from build123d import *

# Parameters (mm, degrees)
F1_DEPTH = 60.325
F2_R     = 6.35
F3_R     = 6.35
F4_W     = 17.4625
F4_H     = 17.4625
F5_DEPTH = 25.4


with BuildPart() as f1:
    # F0 (on Front) → F1 (new body)
    with BuildSketch(Plane.XZ):
        with BuildLine():
            ThreePointArc((18.421305, 15.875), (-31.178134, 43.737725), (-67.557349, 0))
            Line((-67.557349, 0), (-51.682349, 0))
            ThreePointArc((-51.682349, 0), (-23.107349, 28.575), (5.467651, 0))
            Line((5.467651, 0), (65.792651, 0))
            Line((65.792651, 0), (65.792651, 57.15))
            Line((65.792651, 57.15), (49.917651, 57.15))
            Line((49.917651, 57.15), (49.917651, 15.875))
            Line((49.917651, 15.875), (18.421305, 15.875))
        make_face()
    extrude(amount=F1_DEPTH)

    # F2
    f2_edges = [f1.edges().sort_by_distance(p)[0] for p in [
        (57.855151, -60.325, 57.15),
    ]]
    fillet(f2_edges, radius=F2_R)

    # F3
    f3_edges = [f1.edges().sort_by_distance(p)[0] for p in [
        (57.855151, 0, 57.15),
    ]]
    fillet(f3_edges, radius=F3_R)

    # F4 (on face) → F5 (cut)
    with BuildSketch(Plane.YZ.offset(65.792651)):
        with Locations((-31.080982, 48.41875)):
            Rectangle(F4_W, F4_H)
        with BuildLine():
            Line((-22.349732, 39.6875), (-39.812232, 39.6875))
            ThreePointArc((-39.812232, 39.6875), (-31.080982, 30.95625), (-22.349732, 39.6875))
        make_face()
    extrude(amount=-F5_DEPTH, mode=Mode.SUBTRACT)


solid = f1.part
Check sheet for the modelled part. Datum: model origin and axes. Units: mm. A direction names the side the tool comes from. Round coordinates to 2 decimals unless told otherwise and drop trailing zeros. Write each loop counter-clockwise with the first axis right and the second up, starting at its lowest first coordinate (ties: lowest second). Pieces come first, ordered by that corner, then holes. Notation, with made-up numbers: (35.25, -6.5) - (65.25, -6.5) arc R11 cw to (65.25, 12.5) - close; hole circle Ø8 at (78, 74). An arc over 180 degrees is marked (long way). Return JSON: item names as keys, results as strings.
Q1. Cross-section at B-B (y = -44). Record the boundary of the cut face in (x, z) (3 decimals), then the cut area to 3 significant figures.
Returned:
{"outline": "(-67.557, 0) - (-51.682, 0) arc R28.575 cw to (5.468, 0) - (65.793, 0) - (65.793, 57.15) - (49.918, 57.15) - (49.918, 15.875) - (18.421, 15.875) arc R44.45 ccw to start", "area": "3,200 mm²"}
Q2. Draft check along Y on faces 1 (the cylindrical face through (57.74, -1.91, 55.34)), 2 (the cylindrical face through (57.744, -58.415, 55.339)), 3 (the flat face through (58, -39.812, 48)), 4 (the flat face through (35, -30, 0)). Enter one of: released by +Y, released by -Y, zero draft, split by the parting line, or undercut.
Returned:
{"face 1": "released by +Y", "face 2": "released by -Y", "face 3": "undercut", "face 4": "zero draft"}
Q3. Depth check by flat-ended pin: P1, Ø3, axis at x = -34.5, z = 26, coming from the +Y side; P2, Ø4, axis at y = -36, z = 9, coming from the -X side; P3, Ø5, axis at x = -53, y = -34, coming from the +Z side; P4, Ø10, axis at y = -53.5, z = 20, coming from the -X side. Enter the tip coordinate at first touch or a pass-through.
Returned:
{"P1": "stops at y = 0", "P2": "stops at x = -67.01", "P3": "stops at z = 35.03", "P4": "stops at x = -64.96"}
Q4. Cross-section at A-A (z = 48.5). Record the boundary of the cut face in (x, y) (3 decimals), then the cut area to 3 significant figures.
Returned:
{"outline": "(49.918, -60.325) - (65.793, -60.325) - (65.793, -39.812) - (49.918, -39.812) - close; (49.918, -22.35) - (65.793, -22.35) - (65.793, 0) - (49.918, 0) - close", "area": "680 mm²"}
Q5. Cross-section at D-D (z = 19.5). Record the boundary of the cut face in (x, y) (3 decimals).
Returned:
{"outline": "(-63.065, -60.325) - (-43.995, -60.325) - (-43.995, 0) - (-63.065, 0) - close; (-2.22, -60.325) - (16.85, -60.325) - (16.85, 0) - (-2.22, 0) - close; (49.918, -60.325) - (65.793, -60.325) - (65.793, 0) - (49.918, 0) - close"}
Q6. Access from +Z, -Z, +X, -X, +Y, -Y to the whole of each face (thin tool, end or side, straight path). Record for faces 5 (the flat face through (-2, 0, 20)), 6 (the flat face through (58, -22.35, 48)), 7 (the flat face through (34, -30, 15.875)).
Returned:
{"face 5": "+Z, -Z, +X, -X, +Y", "face 6": "+Z, +X", "face 7": "+Z, +Y, -Y"}
Q7. Scan lines: L1, parallel to X at y = -6, z = 22; L2, parallel to X at y = -19, z = 23; L3, parallel to X at y = -20.5, z = 46.5. Record each from-to range of solid material in increasing order. Write a range as from..to.
Returned:
{"L1": "x = -61.75..-41.34, -4.87..15.53, 49.92..65.79", "L2": "x = -61.16..-40.06, -6.15..14.95, 49.92..65.79", "L3": "x = 49.92..65.79"}
